Here's how the part is built. I have some questions about the finished solid (model axes, mm). A direction names the side the tool comes from. Coordinates: 2 decimals unless noted, no trailing zeros. Write each loop counter-clockwise with the first axis right and the second up, starting at its lowest first coordinate (ties: lowest second). Pieces come first, ordered by that corner, then holes. Notation, with made-up numbers: (15.5, -25.5) - (73.5, -25.5) arc R29 cw to (73.5, 3.5) - close; hole circle Ø2 at (10, 30.5). An arc over 180 degrees is marked (long way). Answer in a Markdown table with one row per item. Add a question column.
Item 1: Which directions (+Z, -Z, +X, -X, +Y, -Y) give clear straight access to the entire face, cutting with the end or side of a thin tool? Please do faces 1 (the face through (-27, 15, -1)), 2 (the face through (27, 15, -1)), 3 (the face through (-27.5, 0, -15)).
Item 2: If I drill on probe 1 along Y at (x, z) = (28.15, -32.5); probe 2 along X at (y, z) = (0.5, -8.5); probe 3 along Z at (x, y) = (16, 13.5), over which ranges is the centre line in solid material (lowest first)? Write a range as from..to.
Item 3: Imagine slicing it at C-C (y = 12). Please give me the cut outline in (x, z), plus the area to 3 significant figures.
Item 4: We'd pull the mould along Y, two halves only. Please class faces 4 (the face through (0, -15, -1)), 5 (the face through (28.8, 0.7, -34.4)), 6 (the face through (-28.732, 5.433, -17.71)): +Y half, -Y half, draft (parallel to the pull), parting line (faces both ways), or undercut.
Item 5: Imagine slicing it at A-A (z = -19). Please give me the cut outline in (x, y), plus the area to 3 significant figures.
Item 6: I'm going to push flat-ended pins straight in: pin 1 (2.5 mm diameter, centred on y = 0.07, z = -32.5, fed in from +X); pin 2 (0.8 mm diameter, centred on x = 27, z = -1, fed in from +Y); pin 3 (17.5 mm diameter, centred on x = -5, y = 4.5, fed in from -Z); pin 4 (0.8 mm diameter, centred on y = 18.5, z = -1, fed in from -X). Where does each tip first touch, or does it pass through?
Item 7: Imagine slicing it at D-D (z = -24). Please give me the cut outline in (x, y).
Item 8: Imagine slicing it at B-B (x = 10). Please give me the cut outline in (y, z), plus the area to 3 significant figures.
from build123d import *

# Parameters (mm, degrees)
SALIENTE_EXTRUIR1_DEPTH = 2.5
REDONDEO1_R             = 1
REDONDEO2_R             = 1
CROQUIS3_W              = 2.5
CROQUIS3_H              = 4.8076308
SALIENTE_EXTRUIR2_DEPTH = 30
SALIENTE_EXTRUIR3_DEPTH = 2.5
SALIENTE_EXTRUIR4_START = -2.5
SALIENTE_EXTRUIR4_DEPTH = 2.5
CROQUIS6_R              = 2
CORTAR_EXTRUIR1_DEPTH   = 100


with BuildPart() as part:
    # Croquis2 → Saliente-Extruir1 (new body)
    with BuildSketch(Plane.XY):
        with BuildLine():
            Line((30, -15), (-30, -15))
            Line((-30, -15), (-30, 15))
            Line((-30, 15), (-25, 15))
            ThreePointArc((-25, 15), (-22.878679656, 15.878679656), (-22, 18))
            Line((-22, 18), (-22, 20))
            Line((-22, 20), (22, 20))
            Line((22, 20), (22, 18))
            ThreePointArc((22, 18), (22.878679656, 15.878679656), (25, 15))
            Line((25, 15), (30, 15))
            Line((30, 15), (30, -15))
        make_face()
    extrude(amount=-SALIENTE_EXTRUIR1_DEPTH)

    # Redondeo1
    redondeo1_edges = [part.edges().sort_by_distance(p)[0] for p in [
        (-22, 20, -1.25),
        (22, 20, -1.25),
    ]]
    fillet(redondeo1_edges, radius=REDONDEO1_R)

    # Redondeo2
    redondeo2_edges = [part.edges().sort_by_distance(p)[0] for p in [
        (30, 15, -1.25),
        (30, -15, -1.25),
        (-30, -15, -1.25),
        (-30, 15, -1.25),
    ]]
    fillet(redondeo2_edges, radius=REDONDEO2_R)

    # Croquis3 → Saliente-Extruir2 (add)
    with BuildSketch(Plane(origin=(0, 0, -2.5), x_dir=(-1, 0, 0), z_dir=(0, 0, -1))):
        with Locations((28.75, 0.071092992)):
            Rectangle(CROQUIS3_W, CROQUIS3_H)
        with Locations((-28.75, 0.071092992)):
            Rectangle(CROQUIS3_W, CROQUIS3_H)
    extrude(amount=SALIENTE_EXTRUIR2_DEPTH)

    # Croquis4 → Saliente-Extruir3 (add)
    with BuildSketch(Plane(origin=(30, 0, 0), x_dir=(0, 0, -1), z_dir=(1, 0, 0))):
        with BuildLine():
            Line((32.5, -2.332722408), (2.5, -8.332722408))
            Line((2.5, -8.332722408), (2.5, 2.474908392))
            Line((2.5, 2.474908392), (2.5, 8.474908392))
            Line((2.5, 8.474908392), (32.5, 2.474908392))
            Line((32.5, 2.474908392), (32.5, 2.471092992))
            ThreePointArc((32.5, 2.471092992), (34.9, 0.071092992), (32.5, -2.328907008))
            Line((32.5, -2.328907008), (32.5, -2.332722408))
        make_face()
    extrude(amount=-SALIENTE_EXTRUIR3_DEPTH)

    # Croquis5 → Saliente-Extruir4 (add)
    with BuildSketch(Plane.ZY.offset(30).offset(SALIENTE_EXTRUIR4_START)):
        with BuildLine():
            Line((-2.5, 8.474908392), (-2.5, -8.332722408))
            Line((-2.5, -8.332722408), (-32.5, -2.332722408))
            Line((-32.5, -2.332722408), (-32.5, -2.328907008))
            ThreePointArc((-32.5, -2.328907008), (-34.9, 0.071092992), (-32.5, 2.471092992))
            Line((-32.5, 2.471092992), (-32.5, 2.474908392))
            Line((-32.5, 2.474908392), (-2.5, 8.474908392))
        make_face()
    extrude(amount=SALIENTE_EXTRUIR4_DEPTH)

    # Croquis6 → Cortar-Extruir1 (cut)
    with BuildSketch(Plane(origin=(30, 0, 0), x_dir=(0, 0, -1), z_dir=(1, 0, 0))):
        with Locations((32.5, 0.071092992)):
            Circle(CROQUIS6_R)
    extrude(amount=-CORTAR_EXTRUIR1_DEPTH, mode=Mode.SUBTRACT)


solid = part.part
Here are the results:
| question | item | result |
|---|---|---|
| 1 | face 1 | +Z, -Z, -X, +Y |
| 1 | face 2 | +Z, -Z, +X, +Y |
| 1 | face 3 | -Z, +Y, -Y |
| 2 | probe 1 | y = -2.33..-1.93, 2.07..2.47 |
| 2 | probe 2 | x = -30..-27.5, 27.5..30 |
| 2 | probe 3 | z = -2.5..0 |
| 3 | outline | (-30, -2.5) - (30, -2.5) - (30, 0) - (-30, 0) - close |
| 3 | area | 150 mm2 |
| 4 | face 4 | -Y half |
| 4 | face 5 | undercut |
| 4 | face 6 | +Y half |
| 5 | outline | (-30, -5.03) - (-27.5, -5.03) - (-27.5, 5.17) - (-30, 5.17) - close; (27.5, -5.03) - (30, -5.03) - (30, 5.17) - (27.5, 5.17) - close |
| 5 | area | 51.0 mm2 |
| 6 | pin 1 | passes through |
| 6 | pin 2 | stops at y = 15 |
| 6 | pin 3 | stops at z = -2.5 |
| 6 | pin 4 | stops at x = -22 |
| 7 | outline | (-30, -4.03) - (-27.5, -4.03) - (-27.5, 4.17) - (-30, 4.17) - close; (27.5, -4.03) - (30, -4.03) - (30, 4.17) - (27.5, 4.17) - close |
| 8 | outline | (-15, -2.5) - (20, -2.5) - (20, 0) - (-15, 0) - close |
| 8 | area | 87.5 mm2 |
